For this review, take the finished solid that the model builds, in its own axes (mm). A direction names the side the tool comes from. Round coordinates to 2 decimals unless told otherwise and drop trailing zeros. Loops run counter-clockwise (first coordinate to the right, second up) from the corner with the lowest first, then second, coordinate; pieces in that order, holes last.
1. Draft analysis for pull direction Z (two halves, no side actions). For faces 1 (the cylindrical face through (-3.6, 14.59, 0.57)), 2 (the flat face through (-19.45, 5, 5)), 3 (the cylindrical face through (-17.9, 1.5, 5.8)), state which applies: released by +Z, released by -Z, zero draft, split by the parting line, or undercut.
2. Consider section A-A on y = 7.75. State the section outline as (x, z) points.
3. Tool access review of faces 4 (the cylindrical face through (16.55, 12.74, 4.93)), 5 (the flat face through (1, 14, 10)), 6 (the cylindrical face through (2.43, 14.59, 4.4)): name each direction out of +Z, -Z, +X, -X, +Y, -Y from which nothing blocks a thin tool from reaching the whole face with its end or side.
4. Clearance check with flat-ended pins moving along their axes: pin 1 Ø1.1 at (y, z) = (14, 2.5) entering from +X; pin 2 Ø3 at (x, z) = (2, 6.5) entering from -Y; pin 3 Ø0.6 at (x, y) = (0.5, 14.5) entering from -Z. State where each tip first meets the part, or that it passes through.
5. Consider section B-B on x = 6.5. State the section outline as (y, z) points, then the cut area to 3 significant figures.
6. To check wall thickness, follow line 1 along Z through (x, y) = (6.5, 14.35); line 2 along X through (y, z) = (14.65, 2); line 3 along X through (y, z) = (9.25, 1.5). State the ranges of each line that lie inside material, in increasing order.
7. Consider section D-D on z = 9. State the section outline as (x, y) points, then the cut area to 3 significant figures.
8. Consider section C-C on y = 2.1. State the section outline as (x, z) points, then the cut area to 3 significant figures.
from build123d import *

# Parameters (mm, degrees)
BOSS_EXTRUDE1_DEPTH     = 10
SKETCH2_R               = 1
CUT_EXTRUDE1_DEPTH      = 1
CUT_EXTRUDE1_DEPTH_BACK = 39.9
CHAMFER1_SIZE           = 1
SKETCH3_R               = 0.9
SKETCH3_W               = 6
SKETCH3_H               = 5
CUT_EXTRUDE2_DEPTH      = 16.6
FILLET1_R               = 2


with BuildPart() as part:
    # Sketch1 → Boss-Extrude1 (new body)
    with BuildSketch(Plane.XY):
        with BuildLine():
            Line((17.45, 0), (19.45, 0))
            Line((19.45, 0), (19.45, 10.6))
            ThreePointArc((19.45, 10.6), (17.985533906, 14.135533906), (14.45, 15.6))
            Line((14.45, 15.6), (-14.45, 15.6))
            ThreePointArc((-14.45, 15.6), (-17.985533906, 14.135533906), (-19.45, 10.6))
            Line((-19.45, 10.6), (-19.45, 0))
            Line((-19.45, 0), (-17.45, 0))
            Line((-17.45, 0), (-17.45, 10.6))
            ThreePointArc((-17.45, 10.6), (-16.571320344, 12.721320344), (-14.45, 13.6))
            Line((-14.45, 13.6), (14.45, 13.6))
            ThreePointArc((14.45, 13.6), (16.571320344, 12.721320344), (17.45, 10.6))
            Line((17.45, 10.6), (17.45, 0))
        make_face()
    extrude(amount=BOSS_EXTRUDE1_DEPTH)

    # Sketch2 → Cut-Extrude1 (cut, two sides)
    with BuildSketch(Plane(origin=(19.45, 0, 0), x_dir=(0, 0, -1), z_dir=(1, 0, 0))) as cut_extrude1_sk:
        with Locations((-5, 2.1)):
            Circle(SKETCH2_R)
    extrude(amount=CUT_EXTRUDE1_DEPTH, mode=Mode.SUBTRACT)
    extrude(cut_extrude1_sk.sketch, amount=-CUT_EXTRUDE1_DEPTH_BACK, mode=Mode.SUBTRACT)

    # Chamfer1
    chamfer1_edges = [part.edges().sort_by_distance(p)[0] for p in [
        (-19.45, 2.1, 6),
        (19.45, 2.1, 6),
    ]]
    chamfer(chamfer1_edges, length=CHAMFER1_SIZE)

    # Sketch3 → Cut-Extrude2 (cut, through all)
    with BuildSketch(Plane(origin=(0, 15.6, 0), x_dir=(1, 0, 0), z_dir=(0, 1, 0))):
        with Locations((-6.5, -2)):
            Circle(SKETCH3_R)
        with Locations((6.5, -2)):
            Circle(SKETCH3_R)
        with Locations((0, -2.5)):
            Rectangle(SKETCH3_W, SKETCH3_H)
    extrude(amount=-CUT_EXTRUDE2_DEPTH, mode=Mode.SUBTRACT)

    # Fillet1
    fillet1_edges = [part.edges().sort_by_distance(p)[0] for p in [
        (-3, 14.6, 0),
        (3, 14.6, 0),
        (3, 14.6, 5),
        (-3, 14.6, 5),
    ]]
    fillet(fillet1_edges, radius=FILLET1_R)


solid = part.part
Resolved:
1. face 1: released by -Z
1. face 2: zero draft
1. face 3: undercut
2. outline: (-19.45, 0) - (-17.45, 0) - (-17.45, 10) - (-19.45, 10) - close; (17.45, 0) - (19.45, 0) - (19.45, 10) - (17.45, 10) - close
3. face 4: +Z, -Z, -Y
3. face 5: +Z, +X, -X, +Y, -Y
3. face 6: -Z, +Y, -Y
4. pin 1: stops at x = 18.56
4. pin 2: stops at y = 13.6
4. pin 3: stops at z = 5
5. outline: (13.6, 0) - (15.6, 0) - (15.6, 1.1) - (13.6, 1.1) - close; (13.6, 2.9) - (15.6, 2.9) - (15.6, 10) - (13.6, 10) - close
5. area: 16.4 mm2
6. line 1: z = 0 to 1.1, 2.9 to 10
6. line 2: x = -17.38 to -7.4, -5.6 to -3, 3 to 5.6, 7.4 to 17.38
6. line 3: x = -19.45 to -17.45, 17.45 to 19.45
7. outline: (-19.45, 0) - (-17.45, 0) - (-17.45, 10.6) arc R3 cw to (-14.45, 13.6) - (14.45, 13.6) arc R3 cw to (17.45, 10.6) - (17.45, 0) - (19.45, 0) - (19.45, 10.6) arc R5 ccw to (14.45, 15.6) - (-14.45, 15.6) arc R5 ccw to (-19.45, 10.6) - close
7. area: 125 mm2
8. outline: (-19.45, 0) - (-17.45, 0) - (-17.45, 4) - (-18.45, 4) - (-19.45, 3) - close; (-19.45, 7) - (-18.45, 6) - (-17.45, 6) - (-17.45, 10) - (-19.45, 10) - close; (17.45, 0) - (19.45, 0) - (19.45, 3) - (18.45, 4) - (17.45, 4) - close; (17.45, 6) - (18.45, 6) - (19.45, 7) - (19.45, 10) - (17.45, 10) - close
8. area: 30.0 mm2
